Input: part model. Units: mm. Frame: model coordinates. Face numbers are marked on the shaded views. Give positions to 0.01 mm unless a question says otherwise; leave off trailing zeros. Loops run counter-clockwise (first coordinate to the right, second up) from the corner with the lowest first, then second, coordinate; pieces in that order, holes last. Notation, with made-up numbers: M -9,72 L 34,72 A27 ccw 34,107 Z; hole C 50,46 d9. An arc over 180 degrees is marked long. Use a Markdown table: item, result. Add a question column.
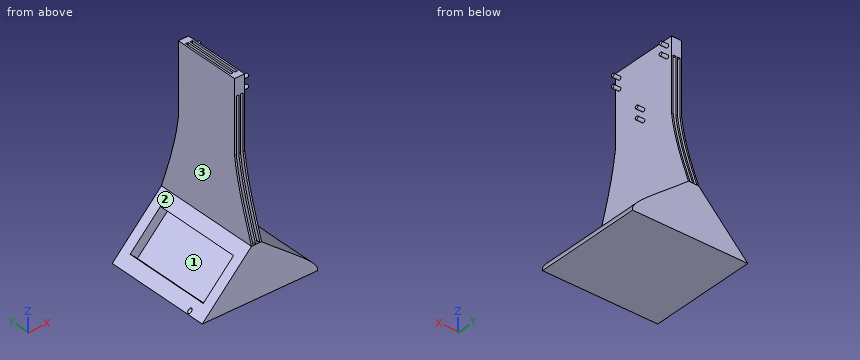
from build123d import *

# Parameters (mm, degrees)
F1_DEPTH  = 320
F2_W      = 30
F2_H      = 320
F3_DEPTH  = 428
F5_DEPTH  = 205
F7_W      = 260
F7_H      = 128.6325914682
F8_DEPTH  = 30
F9_W      = 7.5
F9_H      = 457.219858036
F10_DEPTH = 977
F6_W      = 20
F6_H      = 50
F6_H_2    = 25
F11_DEPTH = 25
F12_R     = 5.1978686685
F13_DEPTH = 63
F14_R     = 5
F15_DEPTH = 20


with BuildPart() as f1:
    # F0 (on Front) → F1 (new body)
    with BuildSketch(Plane.XZ):
        with BuildLine():
            Line((150.299176857, 1.1440683747), (180.299176857, 1.1440683747))
            Line((180.299176857, 1.1440683747), (340.299176857, 1.1440683747))
            add(Edge.make_bspline(
                [(340.299176857, 1.1440683747), (349.1569172885, 24.1151609846), (251.1032390966, 88.0444564268), (175.3079980464, 151.1440683747)],
                knots=[0.4586039165, 0.4586039165, 0.4586039165, 0.4586039165, 1, 1, 1, 1], degree=3))
            Line((175.3079980464, 151.1440683747), (145.3079980464, 151.1440683747))
            Line((145.3079980464, 151.1440683747), (0.299176857, 1.1440683747))
            Line((0.299176857, 1.1440683747), (100.299176857, 1.1440683747))
            Line((100.299176857, 1.1440683747), (150.299176857, 1.1440683747))
        make_face()
    extrude(amount=F1_DEPTH)

    # F2 (on face) → F3 (join)
    with BuildSketch(Plane.XY.offset(151.1440683747)):
        with Locations((160.3079980464, -160)):
            Rectangle(F2_W, F2_H)
    extrude(amount=F3_DEPTH)

    # F4 (on face) → F5 (cut)
    with BuildSketch(Plane(origin=(145.3079980464, 0, 0), x_dir=(0, -1, 0), z_dir=(-1, 0, 0))):
        with BuildLine():
            Line((0, 579.1440683747), (0, 151.1440683747))
            add(Edge.make_bspline(
                [(60, 368.6685562134), (50.1739969339, 296.0916949665), (25.086998467, 223.6178816706), (0, 151.1440683747)],
                knots=[0.4913001533, 0.4913001533, 0.4913001533, 0.4913001533, 1, 1, 1, 1], degree=3))
            Line((60, 368.6685562134), (60, 579.1440683747))
            Line((60, 579.1440683747), (0, 579.1440683747))
        make_face()
        with BuildLine():
            add(Edge.make_bspline(
                [(320, 151.1440683747), (294.913001533, 223.6178816706), (269.8260030661, 296.0916949665), (260, 368.6685562134)],
                knots=[0, 0, 0, 0, 0.5086998467, 0.5086998467, 0.5086998467, 0.5086998467], degree=3))
            Line((320, 151.1440683747), (320, 579.1440683747))
            Line((320, 579.1440683747), (260, 579.1440683747))
            Line((260, 579.1440683747), (260, 368.6685562134))
        make_face()
    extrude(amount=-F5_DEPTH, mode=Mode.SUBTRACT)

    # F7 (on face) → F8 (cut)
    with BuildSketch(Plane(origin=(-0.4170581217, 0, 0.4031807106), x_dir=(0, -1, 0), z_dir=(-0.7189672474, 0, 0.6950439534))):
        with Locations((160, 105.3467844897)):
            Rectangle(F7_W, F7_H)
    extrude(amount=-F8_DEPTH, mode=Mode.SUBTRACT)

    # F9 (on face) → F10 (cut)
    with BuildSketch(Plane.XZ.offset(320)):
        with Locations((154.0579980464, 379.7539973927)):
            Rectangle(F9_W, F9_H)
        with Locations((166.5579980464, 379.7539973927)):
            Rectangle(F9_W, F9_H)
    extrude(amount=-F10_DEPTH, mode=Mode.SUBTRACT)

    # F6 (on face) → F11 (join)
    with BuildSketch(Plane.YZ.offset(175.3079980464)):
        with Locations((-250, 554.1440683747)):
            Rectangle(F6_W, F6_H)
        with Locations((-70, 554.1440683747)):
            Rectangle(F6_W, F6_H)
        with Locations((-230, 406.1685562134)):
            Rectangle(F6_W, F6_H_2)
        with Locations((-90, 406.1685562134)):
            Rectangle(F6_W, F6_H_2)
    extrude(amount=-F11_DEPTH)

    # F12 (on Right) → F13 (cut)
    with BuildSketch(Plane.YZ):
        with Locations((-268.3978974819, 7.7915792353)):
            Circle(F12_R)
    extrude(amount=F13_DEPTH, mode=Mode.SUBTRACT)

    # F14 (on face) → F15 (join)
    with BuildSketch(Plane.YZ.offset(175.3079980464)):
        with Locations((-245, 559.1440683747)):
            Circle(F14_R)
        with Locations((-245, 529.1440683747)):
            Circle(F14_R)
        with Locations((-75, 559.1440683747)):
            Circle(F14_R)
        with Locations((-75, 529.1440683747)):
            Circle(F14_R)
        with Locations((-160, 428.5443711281)):
            Circle(F14_R)
        with Locations((-160, 398.5443711281)):
            Circle(F14_R)
    extrude(amount=F15_DEPTH)


solid = f1.part
1) Section query A-A, the plane z = 503.5. Return the cut outline in (x, y), and give its area (3 significant figures).
2) Contact query for flat-ended pins moving along their axis: P1, Ø12, axis at y = -176.5, z = 412, coming from the +X side; P2, Ø8, axis at x = 152.5, z = 402.5, coming from the +Y side; P3, Ø1, axis at y = -123, z = 228, coming from the -X side. Output: stop coordinate, or through.
3) Section query C-C, the plane x = 127. Return the cut outline in (y, z), and give its area (3 significant figures).
4) Ray query, line 1 (X direction, y = -154.5, z = 325.5); line 2 (X direction, y = -255.5, z = 25.5); line 3 (Y direction, x = 88, z = 51). Return the intervals inside material, ascending. Write a range as [from, to].
5) Section query D-D, the plane y = -233.5. State how many separate pieces and enclosed holes the cut face has, and give its area (3 significant figures).
6) Section query B-B, the plane x = 86.5. Return the cut outline in (y, z), and give its area (3 significant figures).
7) Pull-direction query (Z, two-part tool) for the marked faces 1, 2 and 3; classes: pulls with the +Z half, pulls with the -Z half, needs draft (parallel to the pull), parting line crosses it, or undercut.
Entries:
| question | item | result |
|---|---|---|
| 1 | outline | M 145.31,-260 L 150.31,-260 L 150.31,-60 L 145.31,-60 Z; M 157.81,-260 L 162.81,-260 L 162.81,-60 L 157.81,-60 Z; M 170.31,-260 L 175.31,-260 L 175.31,-60 L 170.31,-60 Z |
| 1 | area | 3,000 mm² |
| 2 | P1 | stops at x = 175.31 |
| 2 | P2 | stops at y = -60 |
| 2 | P3 | stops at x = 145.31 |
| 3 | outline | M -320,1.14 L 0,1.14 L 0,132.21 L -320,132.21 Z; hole M -290,89.04 L -30,89.04 L -30,113.21 L -290,113.21 Z |
| 3 | area | 35,700 mm² |
| 4 | line 1 | x = [145.31, 150.31], [157.81, 162.81], [170.31, 175.31] |
| 4 | line 2 | x = [23.84, 32.66], [65.57, 328.82] |
| 4 | line 3 | y = [-320, -290], [-30, 0] |
| 5 | separate pieces | 1 |
| 5 | enclosed holes | 2 |
| 5 | area | 32,200 mm² |
| 6 | outline | M -320,1.14 L 0,1.14 L 0,90.31 L -30,90.31 L -30,47.15 L -290,47.15 L -290,90.31 L -320,90.31 Z |
| 6 | area | 17,300 mm² |
| 7 | face 1 | undercut |
| 7 | face 2 | pulls with the +Z half |
| 7 | face 3 | needs draft |
